CAD build for the part. Positions are in the model's coordinates, mm. A direction names the side the tool comes from. Coordinates: 2 decimals unless noted, no trailing zeros. Order: outer loops, then holes, each group sorted by start corner. A loop starts at its lowest first (then second) coordinate and runs counter-clockwise, first axis right, second up. Notation, with made-up numbers: (14.25, 81) - (57.25, 81) arc R28 cw to (57.25, 100) - close; hole circle Ø4 at (10.5, 9). An arc over 180 degrees is marked (long way). Use one line per item in the form item = value.
```python
from build123d import *

# Parameters (mm, degrees)
SKETCH2_R           = 85
BOSS_EXTRUDE1_DEPTH = 400
SKETCH4_R           = 60
BOSS_EXTRUDE2_DEPTH = 1000


with BuildPart() as part:
    # Sketch1 → Revolve1 (revolve)
    with BuildSketch(Plane.XY):
        with BuildLine():
            Line((150, 85), (150, 0))
            Line((150, 0), (0, 0))
            add(Edge.make_bspline(
                [(0, 0), (-0.012294225, 3.891554312), (-0.027437579, 8.684958126), (0.361573767, 14.085722357), (0.576098453, 16.090496183), (0.782493435, 17.604822189), (0.986227589, 18.854298664), (1.188670863, 19.931536976), (1.390404268, 20.885679324), (1.591698837, 21.746529091), (1.792703864, 22.533746067), (1.993507167, 23.261083862), (2.253808552, 24.139979457), (2.580573656, 25.146175179), (2.983585386, 26.259501153), (3.385879093, 27.271261727), (3.787683439, 28.201566994), (4.189138614, 29.064817448), (4.590335615, 29.871726974), (5.05331092, 30.74778076), (5.583218589, 31.683457084), (6.185429632, 32.669732492), (6.787226927, 33.590624245), (7.451481511, 34.546094958), (8.182770444, 35.530963646), (8.985083876, 36.540013411), (9.850344603, 37.562485558), (10.782608842, 38.595746542), (11.785011743, 39.636928062), (12.851029789, 40.680352273), (13.983960321, 41.72463117), (15.186170623, 42.768194245), (16.387975322, 43.755294725), (17.654380903, 44.743506811), (18.987602276, 45.731471932), (20.389198856, 46.717890971), (21.790522044, 47.657861765), (23.257103599, 48.59836715), (24.790441056, 49.538186318), (26.391587757, 50.476245251), (28.05829275, 51.412163763), (29.791720393, 52.345056651), (31.59268286, 53.274185034), (33.459445798, 54.199628429), (35.392909821, 55.120726442), (37.459746918, 56.067201212), (39.59327023, 57.006562681), (41.860151348, 57.96659169), (44.193707143, 58.917521836), (46.660609333, 59.885320784), (49.260404933, 60.867669295), (51.99403381, 61.861671206), (54.860992187, 62.865616104), (57.794602823, 63.85555089), (60.861539281, 64.853573463), (64.06149587, 65.858380358), (67.461497598, 66.888166734), (70.995135905, 67.920234745), (74.662088876, 68.953918346), (78.462130407, 69.988575944), (82.462197069, 71.040436012), (86.662284614, 72.107100186), (91.062388571, 73.18640193), (95.662505252, 74.276388609), (100.462631288, 75.375305679), (105.462763855, 76.481579791), (110.662900527, 77.593803027), (116.063039296, 78.710717608), (121.663178505, 79.831201671), (127.529872228, 80.967142806), (133.663251007, 82.116215238), (140.063409966, 83.276352633), (145.198462089, 84.177415336), (148.333178957, 84.715838785), (149.39998937, 84.897876633), (149.733326587, 84.954653305), (149.933332963, 84.98866355), (150, 85)],
                knots=[0, 0, 0, 0, 0.061462209, 0.075705788, 0.085548437, 0.093321935, 0.099856333, 0.105553797, 0.110642995, 0.115267654, 0.119524592, 0.123482434, 0.127191759, 0.134010181, 0.140199136, 0.145901384, 0.151215493, 0.156212588, 0.160945789, 0.165455878, 0.171870938, 0.177937368, 0.183716425, 0.189254732, 0.196326298, 0.203099892, 0.209625632, 0.217492532, 0.225090541, 0.232464167, 0.24106462, 0.249438142, 0.257620809, 0.265641058, 0.274822876, 0.28384341, 0.292725747, 0.301488561, 0.311376345, 0.321146599, 0.330814589, 0.341584449, 0.352255608, 0.362840299, 0.374512001, 0.386101174, 0.398765505, 0.411352526, 0.425006218, 0.438588433, 0.453231339, 0.468927603, 0.484557057, 0.501237456, 0.517857889, 0.535527769, 0.554243231, 0.574001115, 0.593705628, 0.614453399, 0.636242373, 0.65907093, 0.682937829, 0.707842151, 0.733783254, 0.760760729, 0.78877436, 0.81782409, 0.847909993, 0.879032247, 0.912262482, 0.946527454, 0.981827786, 0.994656092, 0.99679374, 0.998931275, 1, 1, 1, 1], degree=3))
        make_face()
    revolve(axis=Axis((0, 0, 0), (-1, 0, 0)))

    # Sketch2 → Boss-Extrude1 (add)
    with BuildSketch(Plane(origin=(150, 0, 0), x_dir=(0, 0, -1), z_dir=(1, 0, 0))):
        Circle(SKETCH2_R)
    extrude(amount=BOSS_EXTRUDE1_DEPTH)

    # Loft1: read off the stored shape, not the designer's step
    # Loft1: loft between two sections, ruled curve by curve
    loft1_from = [
        Edge.make_bspline([(660, 21.137943081, 56.153248902), (660, 133.444440886, 13.877362739), (660, 91.168554723, -98.429135065), (660, -21.137943081, -56.153248902), (660, -133.444440886, -13.877362739), (660, -91.168554723, 98.429135065), (660, 21.137943081, 56.153248902)], [0, 0, 0, 0, 0.5, 0.5, 0.5, 1, 1, 1, 1], 3, [1, 0.333333333, 0.333333333, 1, 0.333333333, 0.333333333, 1]),
    ]
    loft1_to = [
        Edge.make_bspline([(550, 45.635427758, 71.710583133), (550, 189.056594025, -19.560272383), (550, 97.785738508, -162.98143865), (550, -45.635427758, -71.710583133), (550, -189.056594025, 19.560272383), (550, -97.785738508, 162.98143865), (550, 45.635427758, 71.710583133)], [0, 0, 0, 0, 0.5, 0.5, 0.5, 1, 1, 1, 1], 3, [1, 0.333333333, 0.333333333, 1, 0.333333333, 0.333333333, 1]),
    ]
    loft1 = Solid(Shell([*[Face.make_surface_from_curves(loft1_from[k], loft1_to[k]) for k in range(1)], Face(Wire(loft1_from)), Face(Wire(loft1_to))]))
    add(loft1)

    # Sketch4 → Boss-Extrude2 (add)
    with BuildSketch(Plane(origin=(660, 0, 0), x_dir=(0, 0, -1), z_dir=(1, 0, 0))):
        with Locations(Location((0, 0, 0), (0, 0, 159.372))):
            Circle(SKETCH4_R)
    extrude(amount=BOSS_EXTRUDE2_DEPTH)


solid = part.part
```
Item 1: Cut at B-B, the plane x = 1194. Write the cut outline in (y, z), plus the area to 3 significant figures.
Derived:
outline = circle Ø120 at (0, 0)
area = 11,300 mm²
Item 2: Drill centre lines: line 1 (Y direction, x = 288.5, z = -1); line 2 (Y direction, x = 852, z = 0); line 3 (Z direction, x = 329, y = 75). Where is each one in solid material? Low to high. Write a range as [from, to].
Derived:
line_1 = [-84.99, 84.99]
line_2 = [-60, 60]
line_3 = [-40, 40]
Item 3: Cut at A-A, the plane x = 471.5. Write the cut outline in (y, z).
Derived:
outline = circle Ø170 at (0, 0)
Item 4: Drop flat-ended pins along their axis: pin 1 (1 mm diameter, centred on x = 983, y = -22, fed in from -Z); pin 2 (1.5 mm diameter, centred on x = 913.5, y = -3, fed in from +Z); pin 3 (4 mm diameter, centred on y = -25, z = -8.5, fed in from -X). Give the stop position or say it passes through.
Derived:
pin_1 = -56.02
pin_2 = 59.96
pin_3 = 2.34
Item 5: 3-axis set-ups, long thin cutter, end or side, ignore diameter. For faces 1 (the face through (1153, 41.03, 43.78)), 2 (the face through (1660, -1, 0)): which of +Z, -Z, +X, -X, +Y, -Y reach the whole face in a straight line?
Derived:
face_1 = +X
face_2 = +Z, -Z, +X, +Y, -Y
